Could you check a few things on this drawing? It's one solid part, dimensions in mm from its lowest x, y, z. A direction names the side the tool comes from. Coordinates: 2 decimals unless noted, no trailing zeros. Order: outer loops, then holes, each group sorted by start corner. A loop starts at its lowest first (then second) coordinate and runs counter-clockwise, first axis right, second up. Notation, with made-up numbers: M 68.25,67.25 L 81.25,67.25 A24 cw 81.25,85.25 Z; hole C 60,-14.75 d2. An arc over 180 degrees is marked long. Answer as CSV lines item,"result". Start each with the question number.
1. If we mould it in two halves opening along X, with no side actions, what happens to the marked faces 5, 6 and 7? For each: released by +X, released by -X, zero draft, split by the parting line, or undercut.
2. If we section it at C-C (y = 27.5): List the corners of the cut face in (x, z) for me.
3. Will these pins go through, and if not, where does the flat tip stop? pin 1 (14 mm diameter, centred on y = 22, z = 21.5, fed in from -X); pin 2 (14 mm diameter, centred on y = 39.5, z = 24, fed in from +X); pin 3 (16 mm diameter, centred on x = 6, y = 41, fed in from +Z).
4. If we section it at D-D (x = 44): List the corners of the cut face in (y, z) for me.
5. On a 3-axis mill with a long thin cutter (end or side, diameter ignored), from which of +Z, -Z, +X, -X, +Y, -Y can I reach the whole of each face in a straight line? I mean the marked faces 1, 2, 3 and 4. Say none if no direction works.
6. If we section it at B-B (x = 10): List the corners of the cut face in (y, z) for me, plus the area to 3 significant figures.
7. I need wall thicknesses on line 1 along X through (y, z) = (43, 3); line 2 along Y through (x, z) = (85, 1.65); line 3 along X through (y, z) = (44.5, 24.5). Which ranges of each line are inside material? Lowest first, please. Write a range as from..to.
8. If we section it at A-A (z = 17.5): List the corners of the cut face in (x, y) for me, plus the area to 3 significant figures.
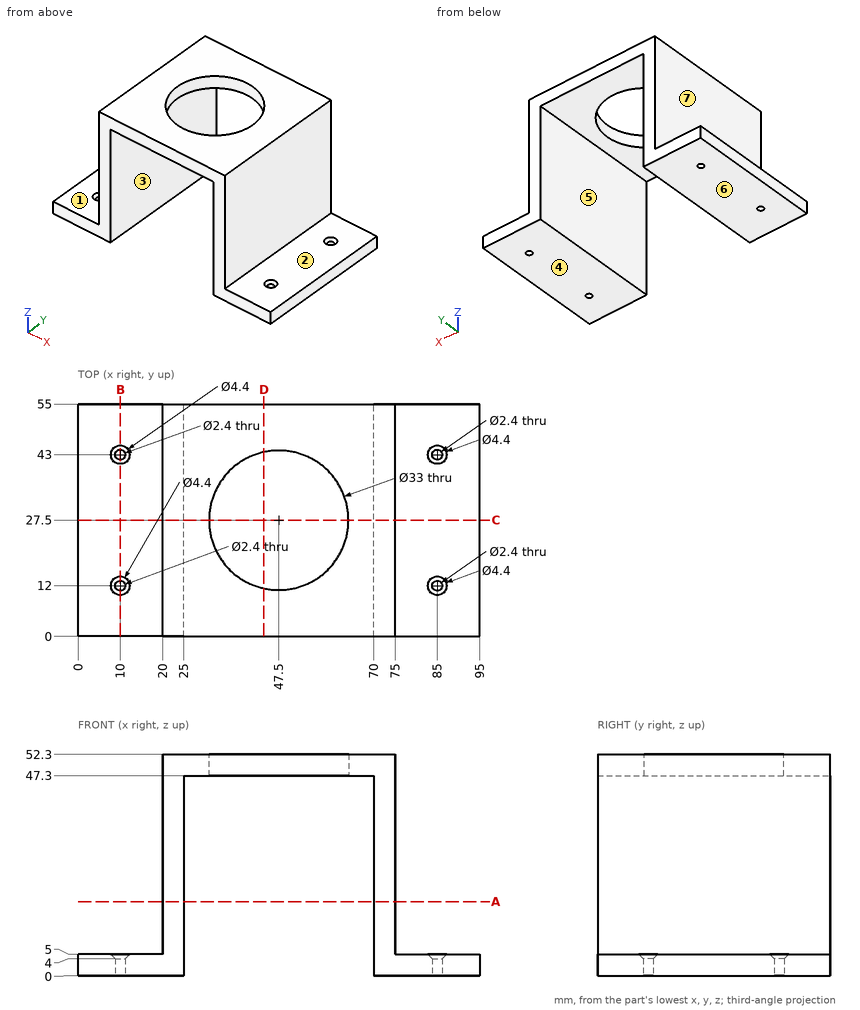
Solved:
1,face 5,"undercut"
1,face 6,"zero draft"
1,face 7,"released by -X"
2,outline,"M 0,0 L 25,0 L 25,47.3 L 31,47.3 L 31,52.3 L 20,52.3 L 20,5 L 0,5 Z; M 64,47.3 L 70,47.3 L 70,0 L 95,0 L 95,5 L 75,5 L 75,52.3 L 64,52.3 Z"
3,pin 1,"x = 20"
3,pin 2,"x = 75"
3,pin 3,"z = 5"
4,outline,"M 0,47.3 L 11.38,47.3 L 11.38,52.3 L 0,52.3 Z; M 43.62,47.3 L 55,47.3 L 55,52.3 L 43.62,52.3 Z"
5,face 1,"+Z, -X, +Y, -Y"
5,face 2,"+Z, +X, +Y, -Y"
5,face 3,"-Z, +Y, -Y"
5,face 4,"-Z, +X, -X, +Y, -Y"
6,outline,"M 0,0 L 10.8,0 L 10.8,4 L 9.8,5 L 0,5 Z; M 13.2,0 L 41.8,0 L 41.8,4 L 40.8,5 L 14.2,5 L 13.2,4 Z; M 44.2,0 L 55,0 L 55,5 L 45.2,5 L 44.2,4 Z"
6,area,"249 mm²"
7,line 1,"0..8.8, 11.2..25, 70..83.8, 86.2..95"
7,line 2,"0..10.8, 13.2..41.8, 44.2..55"
7,line 3,"20..25, 70..75"
8,outline,"M 20,0 L 25,0 L 25,55 L 20,55 Z; M 70,0 L 75,0 L 75,55 L 70,55 Z"
8,area,"550 mm²"
